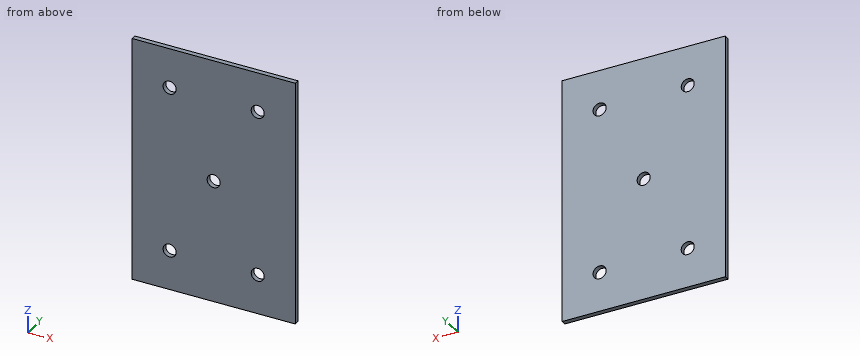
Autodesk Inventor part; units mm, degrees
ref_plane "YZ Plane" through (0, 0, 0) normal (1, 0, 0) x (0, 1, 0)
ref_plane "XZ Plane" through (0, 0, 0) normal (0, 1, 0) x (-1, 0, 0)
ref_plane "XY Plane" through (0, 0, 0) normal (0, 0, 1) x (1, 0, 0)
sketch "Sketch1" plane through (0, 0, 0) normal (0, 1, 0) x (-1, 0, 0)
  line L0 (-50, 75) -> (50, 75)
  line L1 (50, 75) -> (50, -75)
  line L2 (50, -75) -> (-50, -75)
  line L3 (-50, -75) -> (-50, 75)
  circle A0 centre (27, 50.75) radius 4
  line L4 (0, 0) -> (28.2437, 0)
  line L5 (28.2437, 0) -> (0, 0)
  circle A1 centre (27, -50.75) radius 4
  line L6 (0, 0) -> (0, 34.6506)
  circle A2 centre (-27, 50.75) radius 4
  circle A3 centre (-27, -50.75) radius 4
  circle A4 centre (0, 0) radius 4
  point P0 (50, 0)
  point P1 (0, -75)
  dimension "d0" = 101.5
  dimension "d1" = 8
  dimension "d2" = 54
  dimension "d3" = 100
  dimension "d4" = 150
  dimension "d7" = 8
extrude "Extrusion1" add sketch "Sketch1" along normal blind 3
properties part number "PLACA" material "Steel, Mild, Welded"
Model file for the job. Use its own axes, mm. Coordinates: 2 decimals unless noted, no trailing zeros. Order: outer loops, then holes, each group sorted by start corner. A loop starts at its lowest first (then second) coordinate and runs counter-clockwise, first axis right, second up. Notation, with made-up numbers: (69.5, 65) -> (123.5, 65) arc R20 ccw to (123.5, 95) -> close; hole circle Ø9 at (59.25, 30). An arc over 180 degrees is marked (long way). Return JSON: item names as keys, results as strings.
Item 1: Slice it at B-B (y = 1.6). Write the cut outline in (x, z).
Model answer:
{"outline": "(-50, -75) -> (50, -75) -> (50, 75) -> (-50, 75) -> close; hole circle Ø8 at (-27, -50.75); hole circle Ø8 at (-27, 50.75); hole circle Ø8 at (0, 0); hole circle Ø8 at (27, -50.75); hole circle Ø8 at (27, 50.75)"}
Item 2: Pin check, flat tip, straight feed: P1, Ø6.5, axis at x = 27, z = 50.75, coming from the +Y side. Stop position of the tip, or through.
Model answer:
{"P1": "passes through"}
Item 3: Slice it at C-C (z = 0). Write the cut outline in (x, y).
Model answer:
{"outline": "(-50, 0) -> (-4, 0) -> (-4, 3) -> (-50, 3) -> close; (4, 0) -> (50, 0) -> (50, 3) -> (4, 3) -> close"}
Item 4: Slice it at D-D (z = -50.75). Write the cut outline in (x, y), then the cut area to 3 significant figures.
Model answer:
{"outline": "(-50, 0) -> (-31, 0) -> (-31, 3) -> (-50, 3) -> close; (-23, 0) -> (23, 0) -> (23, 3) -> (-23, 3) -> close; (31, 0) -> (50, 0) -> (50, 3) -> (31, 3) -> close", "area": "252 mm²"}
Item 5: Slice it at A-A (x = 27). Write the cut outline in (y, z).
Model answer:
{"outline": "(0, -75) -> (3, -75) -> (3, -54.75) -> (0, -54.75) -> close; (0, -46.75) -> (3, -46.75) -> (3, 46.75) -> (0, 46.75) -> close; (0, 54.75) -> (3, 54.75) -> (3, 75) -> (0, 75) -> close"}
Item 6: Wall check: line 1 along Z through (x, y) = (27, 1.8); line 2 along X through (y, z) = (2, 48.5); line 3 along Z through (x, y) = (0, 1.2). Give the ranges that are in metal, low to high. Write a range as from..to.
Model answer:
{"line 1": "z = -75..-54.75, -46.75..46.75, 54.75..75", "line 2": "x = -50..-30.31, -23.69..23.69, 30.31..50", "line 3": "z = -75..-4, 4..75"}
